```python
from build123d import *

# Parameters (mm, degrees)
SKETCH_1_R          = 22.5
EXTRUDE_1_DEPTH     = 10
SKETCH_2_R          = 2.1
CUT_EXTRUDE_1_DEPTH = 58.445626465
SKETCH_5_R          = 23.6
CUT_EXTRUDE_2_DEPTH = 9


with BuildPart() as part:
    # 草图1 → 凸台-拉伸1 (new body)
    with BuildSketch(Plane(origin=(0, 0, 0), x_dir=(1, 0, 0), z_dir=(0, 1, 0))):
        with BuildLine():
            Line((-40, 0), (-40, -40))
            Line((-40, -40), (40, -40))
            Line((40, -40), (40, 0))
            ThreePointArc((40, 0), (0, 40), (-40, 0))
        make_face()
        with Locations(Location((0, 0, 0), (0, 0, 270))):
            Circle(SKETCH_1_R, mode=Mode.SUBTRACT)
    extrude(amount=EXTRUDE_1_DEPTH)

    # 草图2 → 切除-拉伸1 (cut, through all)
    with BuildSketch(Plane(origin=(0, 10, 0), x_dir=(1, 0, 0), z_dir=(0, 1, 0))):
        with Locations(Location((0, 35, 0), (0, 0, 270))):
            Circle(SKETCH_2_R)
        with Locations(Location((24.748737342, 24.748737342, 0), (0, 0, 270))):
            Circle(SKETCH_2_R)
        with Locations(Location((35, 0, 0), (0, 0, 270))):
            Circle(SKETCH_2_R)
        with Locations(Location((24.748737342, -24.748737342, 0), (0, 0, 270))):
            Circle(SKETCH_2_R)
        with Locations(Location((0, -35, 0), (0, 0, 270))):
            Circle(SKETCH_2_R)
        with Locations(Location((-24.748737342, -24.748737342, 0), (0, 0, 270))):
            Circle(SKETCH_2_R)
        with Locations(Location((-35, 0, 0), (0, 0, 270))):
            Circle(SKETCH_2_R)
        with Locations(Location((-24.748737342, 24.748737342, 0), (0, 0, 270))):
            Circle(SKETCH_2_R)
    extrude(amount=-CUT_EXTRUDE_1_DEPTH, mode=Mode.SUBTRACT)

    # 草图5 → 切除-拉伸2 (cut)
    with BuildSketch(Plane(origin=(0, 10, 0), x_dir=(1, 0, 0), z_dir=(0, 1, 0))):
        with Locations(Location((0, 0, 0), (0, 0, 270))):
            Circle(SKETCH_5_R)
    extrude(amount=-CUT_EXTRUDE_2_DEPTH, mode=Mode.SUBTRACT)


solid = part.part
```
Here's how the part is built. I have some questions about the finished solid (model axes, mm). A direction names the side the tool comes from. Coordinates: 2 decimals unless noted, no trailing zeros. Write each loop counter-clockwise with the first axis right and the second up, starting at its lowest first coordinate (ties: lowest second). Pieces come first, ordered by that corner, then holes. Notation, with made-up numbers: (3.5, 28.25) -> (25.5, 28.25) arc R16 cw to (25.5, 45.25) -> close; hole circle Ø11 at (8.25, 15.5). An arc over 180 degrees is marked (long way). Use a Markdown table: item, result. Add a question column.
(1) For faces 1 (the flat face through (-1, 10, 26)), 2 (the flat face through (-9, 1, 21)), which set-ups out of +Z, -Z, +X, -X, +Y, -Y let a thin tool reach every point of the face, with its end or its side?
(2) If we section it at C-C, the plane x = -13.5: Write out the boundary of the cut face in (y, z), and give its area (3 significant figures).
(3) I'm going to push flat-ended pins straight in: P1, Ø3.5, axis at x = -35, z = 0, coming from the -Y side; P2, Ø2, axis at y = 1.5, z = -3.5, coming from the +X side; P3, Ø10, axis at x = -6.5, z = 16.5, coming from the +Y side. Where does each tip first touch, or does it pass through?
(4) If we section it at D-D, the plane y = 7: State how many separate pieces and enclosed holes the cut face has, and give its area (3 significant figures).
(5) If we section it at A-A, the plane z = 35: Write out the boundary of the cut face in (x, y).
(6) If we section it at B-B, the plane x = 0: Write out the boundary of the cut face in (y, z).
(7) We'd pull the mould along Z, two halves only. Please class faces 3 (the flat face through (-1, 5, 40)), 4 (the cylindrical face through (0.09, 5.07, -37.1)), 5 (the cylindrical face through (0.88, 4.93, -39.99)): +Z half, -Z half, draft (parallel to the pull), parting line (faces both ways), or undercut.
(8) Please list where these lines run through material, in increasing order: line 1 (X direction, y = 7.5, z = 0); line 2 (Z direction, x = -5.5, y = 7); line 3 (X direction, y = 8, z = -1.5).
Outcome:
| question | item | result |
|---|---|---|
| 1 | face 1 | +Z, -Z, +X, -X, +Y |
| 1 | face 2 | +Y |
| 2 | outline | (0, -37.65) -> (10, -37.65) -> (10, -19.36) -> (1, -19.36) -> (1, -18) -> (0, -18) -> close; (0, 18) -> (1, 18) -> (1, 19.36) -> (10, 19.36) -> (10, 40) -> (0, 40) -> close |
| 2 | area | 392 mm^2 |
| 3 | P1 | passes through |
| 3 | P2 | stops at x = 39.92 |
| 3 | P3 | stops at y = 1 |
| 4 | separate pieces | 1 |
| 4 | enclosed holes | 9 |
| 4 | area | 3,850 mm^2 |
| 5 | outline | (-40, 0) -> (-2.1, 0) -> (-2.1, 10) -> (-40, 10) -> close; (2.1, 0) -> (40, 0) -> (40, 10) -> (2.1, 10) -> close |
| 6 | outline | (0, -40) -> (10, -40) -> (10, -37.1) -> (0, -37.1) -> close; (0, -32.9) -> (10, -32.9) -> (10, -23.6) -> (1, -23.6) -> (1, -22.5) -> (0, -22.5) -> close; (0, 22.5) -> (1, 22.5) -> (1, 23.6) -> (10, 23.6) -> (10, 32.9) -> (0, 32.9) -> close; (0, 37.1) -> (10, 37.1) -> (10, 40) -> (0, 40) -> close |
| 7 | face 3 | +Z half |
| 7 | face 4 | undercut |
| 7 | face 5 | -Z half |
| 8 | line 1 | x = -40 to -37.1, -32.9 to -23.6, 23.6 to 32.9, 37.1 to 40 |
| 8 | line 2 | z = -39.62 to -22.95, 22.95 to 40 |
| 8 | line 3 | x = -39.97 to -36.47, -33.53 to -23.55, 23.55 to 33.53, 36.47 to 39.97 |
